Part model, mm, in its own coordinate system. Coordinates: 2 decimals unless noted, no trailing zeros. Loops run counter-clockwise (first coordinate to the right, second up) from the corner with the lowest first, then second, coordinate; pieces in that order, holes last. Notation, with made-up numbers: M -29,68 L 22,68 A28 cw 22,94 Z; hole C -19.5,-27 d7. An arc over 180 degrees is marked long. Answer as a JSON object with one key per item and string values. Group by question number.
1. Drop flat-ended pins along their axis: pin 1 Ø1.5 at (x, y) = (-5.5, -3.5) entering from -Z; pin 2 Ø1 at (y, z) = (-2, 24) entering from +X; pin 3 Ø12.5 at (x, z) = (0, 70.11) entering from +Y; pin 4 Ø3 at (x, y) = (-29.5, -4) entering from -Z. Give the stop position or say it passes through.
2. Saw through at A-A on z = -30. Write the cut outline in (x, y), then the cut area to 3 significant figures.
3. Drill centre lines: L1, parallel to X at y = -4.75, z = 52; L2, parallel to X at y = -5.25, z = -41.5; L3, parallel to Z at x = 38, y = -3. Where is each one in solid material? Low to high.
4. Saw through at B-B on x = -48. Write the cut outline in (y, z), then the cut area to 3 significant figures.
5. Saw through at D-D on z = 53.5. Write the cut outline in (x, y), then the cut area to 3 significant figures.
6. Saw through at C-C on x = 30. Write the cut outline in (y, z).
from build123d import *

# Parameters (mm, degrees)
F1_DEPTH = 6.35


with BuildPart() as f1:
    # F0 (on Front) → F1 (new body)
    with BuildSketch(Plane.XZ):
        with BuildLine():
            ThreePointArc((-7.8402373447, 61.7634878521), (-41.1586655068, -46.7136169332), (62.2591178325, 0))
            ThreePointArc((62.2591178325, 0), (46.7136169332, 41.1586655068), (7.8402373447, 61.7634878521))
            ThreePointArc((7.8402373447, 61.7634878521), (0, 58.6588690032), (-7.8402373447, 61.7634878521))
        make_face()
        with BuildLine():
            ThreePointArc((55.4505510699, 15.5277837924), (57.0478759304, 7.8368064468), (57.5836407625, 0))
            ThreePointArc((57.5836407625, 0), (51.9864857424, -24.7645105668), (36.2831125051, -44.7147786576))
            ThreePointArc((36.2831125051, -44.7147786576), (35.0774454381, -45.6667111252), (33.8468148135, -46.5861439748))
            ThreePointArc((33.8468148135, -46.5861439748), (32.8818393757, -47.27219397), (31.9029625874, -47.9382588504))
            ThreePointArc((31.9029625874, -47.9382588504), (0.3521951536, -57.582563698), (-31.3141832441, -48.3249170844))
            ThreePointArc((-31.3141832441, -48.3249170844), (-32.5920964338, -47.4724228738), (-33.8468148135, -46.5861439748))
            ThreePointArc((-33.8468148135, -46.5861439748), (-34.7974809413, -45.8803989041), (-35.7334358491, -45.1552571234))
            ThreePointArc((-35.7334358491, -45.1552571234), (-54.6554381422, -18.1289482582), (-55.6363420799, 14.848337396))
            ThreePointArc((-55.6363420799, 14.848337396), (-55.2204687988, 16.3271402609), (-54.7652967791, 17.7943235936))
            ThreePointArc((-54.7652967791, 17.7943235936), (-54.3878653203, 18.9165480298), (-53.987440477, 20.0307751774))
            ThreePointArc((-53.987440477, 20.0307751774), (-34.1311135955, 46.3782574941), (-3.070967171, 57.5016942715))
            ThreePointArc((-3.070967171, 57.5016942715), (-1.5360301586, 57.5631504942), (0, 57.5836407625))
            ThreePointArc((0, 57.5836407625), (1.1839315978, 57.5714685364), (2.3673626687, 57.534957004))
            ThreePointArc((2.3673626687, 57.534957004), (33.5612498663, 46.7922877286), (53.7383799899, 20.6896640745))
            ThreePointArc((53.7383799899, 20.6896640745), (54.2711499531, 19.248843244), (54.7652967791, 17.7943235936))
            ThreePointArc((54.7652967791, 17.7943235936), (55.1195752881, 16.6645763079), (55.4505510699, 15.5277837924))
        make_face(mode=Mode.SUBTRACT)
        with BuildLine():
            ThreePointArc((3.19e-08, 62.2591178325), (3.9279438387, 62.1350867906), (7.8402373447, 61.7634878521))
            ThreePointArc((7.8402373447, 61.7634878521), (10.5103201859, 65.5632316042), (11.4519661318, 70.110835135))
            ThreePointArc((11.4519661318, 70.110835135), (-4.5476035308, 80.6211553209), (-7.8402373447, 61.7634878521))
            ThreePointArc((-7.8402373447, 61.7634878521), (-3.9279438068, 62.1350867926), (3.19e-08, 62.2591178325))
        make_face()
        with BuildLine():
            ThreePointArc((7.8517173025, 70.110835135), (5.5520025598, 64.5588325977), (3.19e-08, 62.2591178325))
            ThreePointArc((3.19e-08, 62.2591178325), (-5.5520025598, 75.6628376722), (7.8517173025, 70.110835135))
        make_face(mode=Mode.SUBTRACT)
        with BuildLine():
            Line((16.1334199845, 17.7943235936), (54.7652967791, 17.7943235936))
            ThreePointArc((54.7652967791, 17.7943235936), (54.2711499531, 19.248843244), (53.7383799899, 20.6896640745))
            Line((53.7383799899, 20.6896640745), (15.1282112975, 20.8753324215))
            Line((15.1282112975, 20.8753324215), (16.1334199845, 17.7943235936))
        make_face()
        with BuildLine():
            ThreePointArc((33.8468148135, -46.5861439748), (35.0774454381, -45.6667111252), (36.2831125051, -44.7147786576))
            Line((36.2831125051, -44.7147786576), (24.5284953147, -7.9369514529))
            Line((24.5284953147, -7.9369514529), (21.9089083593, -9.8450458125))
            Line((21.9089083593, -9.8450458125), (33.8468148135, -46.5861439748))
        make_face()
        with BuildLine():
            Line((-11.9379064542, 20.8425426002), (0, 57.5836407625))
            ThreePointArc((0, 57.5836407625), (-1.5360301586, 57.5631504942), (-3.070967171, 57.5016942715))
            Line((-3.070967171, 57.5016942715), (-15.1787465438, 20.8386164159))
            Line((-15.1787465438, 20.8386164159), (-11.9379064542, 20.8425426002))
        make_face()
        with BuildLine():
            Line((-24.5091925682, -7.9963591979), (-23.5114519277, -4.9129238547))
            Line((-23.5114519277, -4.9129238547), (-54.7652967791, 17.7943235936))
            ThreePointArc((-54.7652967791, 17.7943235936), (-55.2204687988, 16.3271402609), (-55.6363420799, 14.848337396))
            Line((-55.6363420799, 14.848337396), (-24.5091925682, -7.9963591979))
        make_face()
        with BuildLine():
            ThreePointArc((-33.8468148135, -46.5861439748), (-32.5920964338, -47.4724228738), (-31.3141832441, -48.3249170844))
            Line((-31.3141832441, -48.3249170844), (0.0312324998, -25.7806381864))
            Line((0.0312324998, -25.7806381864), (-2.592969962, -23.8788965265))
            Line((-2.592969962, -23.8788965265), (-33.8468148135, -46.5861439748))
        make_face()
        with BuildLine():
            Line((24.5284953147, -7.9369514529), (55.4505510699, 15.5277837924))
            ThreePointArc((55.4505510699, 15.5277837924), (55.1195752881, 16.6645763079), (54.7652967791, 17.7943235936))
            Line((54.7652967791, 17.7943235936), (23.5360472008, -4.8950543427))
            Line((23.5360472008, -4.8950543427), (24.5284953147, -7.9369514529))
        make_face()
        with BuildLine():
            Line((15.1282112975, 20.8753324215), (2.3673626687, 57.534957004))
            ThreePointArc((2.3673626687, 57.534957004), (1.1839315978, 57.5714685364), (0, 57.5836407625))
            Line((0, 57.5836407625), (11.9285118958, 20.8714560779))
            Line((11.9285118958, 20.8714560779), (15.1282112975, 20.8753324215))
        make_face()
        with BuildLine():
            Line((-54.7652967791, 17.7943235936), (-16.1638214141, 17.7943235936))
            Line((-16.1638214141, 17.7943235936), (-15.1787465438, 20.8386164159))
            Line((-15.1787465438, 20.8386164159), (-53.987440477, 20.0307751774))
            ThreePointArc((-53.987440477, 20.0307751774), (-54.3878653203, 18.9165480298), (-54.7652967791, 17.7943235936))
        make_face()
        with BuildLine():
            ThreePointArc((-35.7334358491, -45.1552571234), (-34.7974809413, -45.8803989041), (-33.8468148135, -46.5861439748))
            Line((-33.8468148135, -46.5861439748), (-21.9183029177, -9.8739592902))
            Line((-21.9183029177, -9.8739592902), (-24.5091925682, -7.9963591979))
            Line((-24.5091925682, -7.9963591979), (-35.7334358491, -45.1552571234))
        make_face()
        with BuildLine():
            ThreePointArc((31.9029625874, -47.9382588504), (32.8818393757, -47.27219397), (33.8468148135, -46.5861439748))
            Line((33.8468148135, -46.5861439748), (2.6175652352, -23.8967660385))
            Line((2.6175652352, -23.8967660385), (0.0312324998, -25.7806381864))
            Line((0.0312324998, -25.7806381864), (31.9029625874, -47.9382588504))
        make_face()
        Polygon((23.5360472008, -4.8950543427), (16.1334199845, 17.7943235936), (12.9283328478, 17.7943235936), (20.9184819657, -6.7968268059), align=None)
        Polygon((2.6175652352, -23.8967660385), (21.9089083593, -9.8450458125), (20.9184819657, -6.7968268059), (0, -21.9949935753), align=None)
        Polygon((-12.9283328478, 17.7943235936), (12.9283328478, 17.7943235936), (11.9285118958, 20.8714560779), (-11.9379064542, 20.8425426002), align=None)
        Polygon((-20.9184819657, -6.7968268059), (-12.9283328478, 17.7943235936), (-16.1638214141, 17.7943235936), (-23.5114519277, -4.9129238547), align=None)
        Polygon((-2.592969962, -23.8788965265), (0, -21.9949935753), (-20.9184819657, -6.7968268059), (-21.9183029177, -9.8739592902), align=None)
        with BuildLine():
            ThreePointArc((-7.8402373447, 61.7634878521), (0, 58.6588690032), (7.8402373447, 61.7634878521))
            ThreePointArc((7.8402373447, 61.7634878521), (3.9279438387, 62.1350867906), (3.19e-08, 62.2591178325))
            ThreePointArc((3.19e-08, 62.2591178325), (-3.9279438068, 62.1350867926), (-7.8402373447, 61.7634878521))
        make_face()
        Polygon((21.9089083593, -9.8450458125), (24.5284953147, -7.9369514529), (23.5360472008, -4.8950543427), (20.9184819657, -6.7968268059), align=None)
        Polygon((12.9283328478, 17.7943235936), (16.1334199845, 17.7943235936), (15.1282112975, 20.8753324215), (11.9285118958, 20.8714560779), align=None)
        Polygon((-16.1638214141, 17.7943235936), (-12.9283328478, 17.7943235936), (-11.9379064542, 20.8425426002), (-15.1787465438, 20.8386164159), align=None)
        Polygon((-21.9183029177, -9.8739592902), (-20.9184819657, -6.7968268059), (-23.5114519277, -4.9129238547), (-24.5091925682, -7.9963591979), align=None)
        Polygon((0.0312324998, -25.7806381864), (2.6175652352, -23.8967660385), (0, -21.9949935753), (-2.592969962, -23.8788965265), align=None)
    extrude(amount=F1_DEPTH)


solid = f1.part
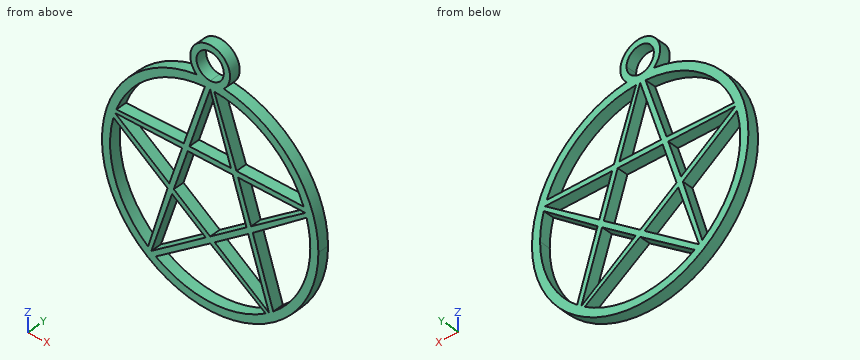
Outcome:
{
 "1": {"pin 1": "stops at z = -62.08", "pin 2": "stops at x = 57.65", "pin 3": "passes through", "pin 4": "stops at z = -55.61"},
 "2": {"outline": "M -54.55,-6.35 L -49.15,-6.35 L -49.15,0 L -54.55,0 Z; M -31.16,-6.35 L -28.46,-6.35 L -28.46,0 L -31.16,0 Z; M -11.02,-6.35 L -5.84,-6.35 L -5.84,0 L -11.02,0 Z; M 6.1,-6.35 L 11.02,-6.35 L 11.02,0 L 6.1,0 Z; M 28.46,-6.35 L 31.58,-6.35 L 31.58,0 L 28.46,0 Z; M 49.15,-6.35 L 54.55,-6.35 L 54.55,0 L 49.15,0 Z", "area": "170 mm²"},
 "3": {"L1": "x = -34.24 to -24.74, -4.89 to -1.81, 1.81 to 4.29, 24.74 to 34.24", "L2": "x = -46.41 to -39.92, -34.63 to -32.19, -26.85 to -21.82, 22.64 to 26.85, 32.19 to 35.26, 39.92 to 46.41", "L3": "z = -49.32 to -43.27, 2.29 to 5.61, 17.79 to 20.77, 43.27 to 49.32"},
 "4": {"outline": "M -6.35,-39.65 L 0,-39.65 L 0,-31.81 L -6.35,-31.81 Z; M -6.35,9.24 L 0,9.24 L 0,12.88 L -6.35,12.88 Z; M -6.35,17.79 L 0,17.79 L 0,20.16 L -6.35,20.16 Z; M -6.35,31.81 L 0,31.81 L 0,39.65 L -6.35,39.65 Z", "area": "138 mm²"},
 "5": {"outline": "M -31.84,-6.35 L -21.3,-6.35 L -21.3,0 L -31.84,0 Z; M -4.39,-6.35 L -1.33,-6.35 L -1.33,0 L -4.39,0 Z; M 1.33,-6.35 L 3.77,-6.35 L 3.77,0 L 1.33,0 Z; M 21.3,-6.35 L 31.84,-6.35 L 31.84,0 L 21.3,0 Z", "area": "169 mm²"},
 "6": {"outline": "M -6.35,-54.55 L 0,-54.55 L 0,-49.15 L -6.35,-49.15 Z; M -6.35,-46.62 L 0,-46.62 L 0,-43.79 L -6.35,-43.79 Z; M -6.35,-34.75 L 0,-34.75 L 0,-25.06 L -6.35,-25.06 Z; M -6.35,-3.78 L 0,-3.78 L 0,-0.2 L -6.35,-0.2 Z; M -6.35,17.79 L 0,17.79 L 0,20.8 L -6.35,20.8 Z; M -6.35,49.15 L 0,49.15 L 0,54.55 L -6.35,54.55 Z"}
}
